Verification items for the finished model (mm, model axes). A direction names the side the tool comes from. Coordinates: 2 decimals unless noted, no trailing zeros. Order: outer loops, then holes, each group sorted by start corner. A loop starts at its lowest first (then second) coordinate and runs counter-clockwise, first axis right, second up.
Q1. Thickness scan on line 1 (Y direction, x = -2, z = 46.5); line 2 (X direction, y = -2, z = 47.5); line 3 (Z direction, x = 25.5, y = 1.25). Record the ranges inside material, lowest first.
Q2. Draft check along Y on faces 4 (the flat face through (29.63, -6.82, 73.93)), 5 (the flat face through (25, 6.16, 74)), 6 (the flat face through (-47, -9.16, 84)). Enter one of: pulls with the +Y half, pulls with the -Y half, needs draft (parallel to the pull), parting line crosses it, or undercut.
Q3. Set-up check for faces 1 (the cylindrical face through (26.366, 7.681, 75.109)), 2 (the flat face through (-35, 6.66, 62)), 3 (the cylindrical face through (-41.348, 7.681, 17.67)): record each of +Z, -Z, +X, -X, +Y, -Y from which the full face is reachable in a straight line by a thin tool's end or side.
Q4. Cross-section at D-D, the plane x = -19.5. Record the boundary of the cut face in (y, z), and give its area (3 significant figures).
Q5. Cross-section at C-C, the plane z = 41.5. Record the boundary of the cut face in (x, y), and give its area (3 significant figures).
Q6. Depth check by flat-ended pin: P1, Ø1.5, axis at x = 1, z = 36.5, coming from the -Y side; P2, Ø4.5, axis at x = 34.5, z = 85, coming from the +Y side; P3, Ø3, axis at x = -5.5, y = 5.5, coming from the +Z side. Enter the tip coordinate at first touch or a pass-through.
Q7. Cross-section at A-A, the plane y = -0.75. Record the boundary of the cut face in (x, z), and give its area (3 significant figures).
Q8. Cross-section at B-B, the plane x = 0. Record the boundary of the cut face in (y, z), and give its area (3 significant figures).
from build123d import *

# Parameters (mm, degrees)
BOSS_EXTRUDE1_DEPTH = 92.4
BOSS_EXTRUDE2_DEPTH = 3
SKETCH3_R           = 1.5
CUT_EXTRUDE1_DEPTH  = 19.319620864
CUT_EXTRUDE2_DEPTH  = 19.319620864


with BuildPart() as part:
    # Sketch1 → Boss-Extrude1 (new body)
    with BuildSketch(Plane.XY):
        Polygon((-52.775, -9.159810432), (-41.775, -9.159810432), (-35.789647492, 6.659810432), (20.684055398, 6.659810432), (26.669407906, -9.159810432), (37.669407906, -9.159810432), (37.669407906, -6.659810432), (28.857556463, -6.659810432), (22.872203955, 9.159810432), (-37.977796049, 9.159810432), (-44.73566716, -6.659810432), (-52.775, -6.659810432), align=None)
    extrude(amount=BOSS_EXTRUDE1_DEPTH)

    # Sketch2 → Boss-Extrude2 (add)
    with BuildSketch(Plane(origin=(0, 9.159810432, 0), x_dir=(1, 0, 0), z_dir=(0, 1, 0))):
        with BuildLine():
            Line((-32.891525537, -77.579025356), (-26.07351169, -71.059265718))
            ThreePointArc((-26.07351169, -71.059265718), (-7.552796047, -77.2), (10.967919597, -71.059265718))
            Line((10.967919597, -71.059265718), (17.785933443, -77.579025356))
            ThreePointArc((17.785933443, -77.579025356), (25.090877354, -77.415674983), (24.927526982, -70.110731072))
            Line((24.927526982, -70.110731072), (18.109513135, -63.590971435))
            ThreePointArc((18.109513135, -63.590971435), (23.447203953, -46.2), (18.109513135, -28.809028565))
            Line((18.109513135, -28.809028565), (24.571212266, -22.629996647))
            ThreePointArc((24.571212266, -22.629996647), (25.083083856, -15.332846234), (17.785933443, -14.820974644))
            Line((17.785933443, -14.820974644), (10.967919597, -21.340734282))
            ThreePointArc((10.967919597, -21.340734282), (-7.552796047, -15.2), (-26.07351169, -21.340734282))
            Line((-26.07351169, -21.340734282), (-32.891525537, -14.820974644))
            ThreePointArc((-32.891525537, -14.820974644), (-40.188675949, -15.332846234), (-39.676804359, -22.629996647))
            Line((-39.676804359, -22.629996647), (-33.215105229, -28.809028565))
            ThreePointArc((-33.215105229, -28.809028565), (-38.552796047, -46.2), (-33.215105229, -63.590971435))
            Line((-33.215105229, -63.590971435), (-40.033119075, -70.110731072))
            ThreePointArc((-40.033119075, -70.110731072), (-40.196469448, -77.415674983), (-32.891525537, -77.579025356))
        make_face()
    extrude(amount=-BOSS_EXTRUDE2_DEPTH)

    # Sketch3 → Cut-Extrude1 (cut, through all)
    with BuildSketch(Plane(origin=(0, 9.159810432, 0), x_dir=(1, 0, 0), z_dir=(0, 1, 0))):
        with Locations((-36.284164948, -18.725485646)):
            Circle(SKETCH3_R)
        with Locations((21.178572854, -18.725485646)):
            Circle(SKETCH3_R)
        with Locations((-36.462322306, -73.844878214)):
            Circle(SKETCH3_R)
        with Locations((21.356730213, -73.844878214)):
            Circle(SKETCH3_R)
    extrude(amount=-CUT_EXTRUDE1_DEPTH, mode=Mode.SUBTRACT)

    # Sketch4 → Cut-Extrude2 (cut, through all)
    with BuildSketch(Plane(origin=(0, 9.159810432, 0), x_dir=(1, 0, 0), z_dir=(0, 1, 0))):
        with BuildLine():
            Line((-44.73566716, -6.607100908), (-36.284164948, -13.552941945))
            ThreePointArc((-36.284164948, -13.552941945), (-34.473232239, -13.880309585), (-32.891525537, -14.820974644))
            Line((-32.891525537, -14.820974644), (-26.99023083, -20.464117047))
            ThreePointArc((-26.99023083, -20.464117047), (-7.552796047, -13.948650534), (11.884638737, -20.464117047))
            Line((11.884638737, -20.464117047), (17.785933443, -14.820974644))
            ThreePointArc((17.785933443, -14.820974644), (19.367640146, -13.880309585), (21.178572854, -13.552941945))
            Line((21.178572854, -13.552941945), (28.857556463, -7.241992941))
            Line((28.857556463, -7.241992941), (28.857556463, 0))
            Line((28.857556463, 0), (-44.73566716, 0))
            Line((-44.73566716, 0), (-44.73566716, -6.607100908))
        make_face()
        with BuildLine():
            Line((28.857556463, -85.158007059), (21.178572854, -78.847058055))
            ThreePointArc((21.178572854, -78.847058055), (19.367640146, -78.519690415), (17.785933443, -77.579025356))
            Line((17.785933443, -77.579025356), (11.884638737, -71.935882953))
            ThreePointArc((11.884638737, -71.935882953), (-7.552796047, -78.451349466), (-26.99023083, -71.935882953))
            Line((-26.99023083, -71.935882953), (-32.891525537, -77.579025356))
            ThreePointArc((-32.891525537, -77.579025356), (-34.473232239, -78.519690415), (-36.284164948, -78.847058055))
            Line((-36.284164948, -78.847058055), (-44.73566716, -85.792899092))
            Line((-44.73566716, -85.792899092), (-44.73566716, -92.4))
            Line((-44.73566716, -92.4), (28.857556463, -92.4))
            Line((28.857556463, -92.4), (28.857556463, -85.158007059))
        make_face()
        with BuildLine():
            Line((-39.676804359, -22.629996647), (-52.775, -11.865284942))
            Line((-52.775, -11.865284942), (-52.775, -80.534715058))
            Line((-52.775, -80.534715058), (-39.676804359, -69.770003353))
            Line((-39.676804359, -69.770003353), (-34.131824369, -64.46758867))
            ThreePointArc((-34.131824369, -64.46758867), (-39.804145512, -46.2), (-34.131824369, -27.93241133))
            Line((-34.131824369, -27.93241133), (-39.676804359, -22.629996647))
        make_face()
        with BuildLine():
            Line((24.571212266, -69.770003353), (37.669407906, -80.534715058))
            Line((37.669407906, -80.534715058), (37.669407906, -11.865284942))
            Line((37.669407906, -11.865284942), (24.571212266, -22.629996647))
            Line((24.571212266, -22.629996647), (19.026232275, -27.93241133))
            ThreePointArc((19.026232275, -27.93241133), (24.698553419, -46.2), (19.026232275, -64.46758867))
            Line((19.026232275, -64.46758867), (24.571212266, -69.770003353))
        make_face()
    extrude(amount=-CUT_EXTRUDE2_DEPTH, mode=Mode.SUBTRACT)


solid = part.part
Check values:
1. line 1: y = 6.16 to 9.16
1. line 2: x = -39.78 to -39.07, 23.96 to 24.67
1. line 3: z = 10 to 21.87, 70.53 to 82.4
2. face 4: needs draft
2. face 5: undercut
2. face 6: pulls with the -Y half
3. face 1: +X, +Y
3. face 2: -Y
3. face 3: -X, +Y
4. outline: (6.16, 17.59) - (6.66, 17.59) - (6.66, 16.24) - (9.16, 16.24) - (9.16, 76.16) - (6.66, 76.16) - (6.66, 74.81) - (6.16, 74.81) - close
4. area: 178 mm2
5. outline: (-39.46, -3.04) - (-35.98, 6.16) - (20.87, 6.16) - (24.35, -3.04) - (24.35, 5.24) - (23.09, 8.59) - (23.09, 9.16) - (-38.19, 9.16) - (-38.19, 8.65) - (-39.46, 5.69) - close
5. area: 218 mm2
6. P1: stops at y = 6.16
6. P2: stops at y = -6.66
6. P3: stops at z = 78.43
7. outline: (-42.21, 8.68) - (-38.59, 11.66) - (-38.59, 23.67) - (-39.68, 22.63) - (-42.21, 20.55) - close; (-42.21, 71.85) - (-39.68, 69.77) - (-38.59, 68.73) - (-38.59, 80.74) - (-42.21, 83.72) - close; (-38.59, 37.45) - (-38.59, 54.95) arc R32.25 ccw to start; (23.49, 11.66) - (26.62, 9.08) - (26.62, 20.94) - (24.57, 22.63) - (23.49, 23.67) - close; (23.49, 37.45) arc R32.25 ccw to (23.49, 54.95) - close; (23.49, 68.73) - (24.57, 69.77) - (26.62, 71.46) - (26.62, 83.32) - (23.49, 80.74) - close
7. area: 189 mm2
8. outline: (6.16, 16.13) - (6.66, 16.13) - (6.66, 14.85) - (9.16, 14.85) - (9.16, 77.55) - (6.66, 77.55) - (6.66, 76.27) - (6.16, 76.27) - close
8. area: 187 mm2
